from build123d import *

# Parameters (mm, degrees)
F0_W        = 50.8
F0_H        = 3.0988
F1_DEPTH    = 8.89
F3_R        = 1.778
F4_T1_DEPTH = 59.9449047052
F5_DEPTH    = 25.4


# Not quite as in the source:
# - a fillet or chamfer that OpenCascade refuses, or shapes differently, is made with other operations: its cross-section is extruded or revolved along the edge and cut away or added


with BuildPart() as f1:
    # F0 (on Top) → F1 (new body)
    with BuildSketch(Plane.XY):
        with Locations((0, 1.5494)):
            Rectangle(F0_W, F0_H)
    extrude(amount=F1_DEPTH)

    # F3
    f3_edges = [f1.edges().sort_by_distance(p)[0] for p in [
        (0, 3.0988, 8.89),
    ]]
    fillet(f3_edges, radius=F3_R)

    # F4: chamfer of 1.778 on 1 edges, made by hand

    # F4_s2 → F4_t1 (cut)
    with BuildSketch(Plane.YZ.offset(-29.9724523526)):
        Polygon((1.778, 8.89), (0, 7.112), (0, 8.89), align=None)
    extrude(amount=F4_T1_DEPTH, mode=Mode.SUBTRACT)

    # F2 (on face) → F5 (cut)
    with BuildSketch(Plane.XZ):
        Polygon((-22.225, 7.8332954744), (-21.6149113577, 8.89), (-22.8350886423, 8.89), align=None)
        Polygon((-12.6515878735, 8.89), (-14.0184121265, 8.89), (-13.335, 7.7062954744), align=None)
        Polygon((14.2383825791, 8.89), (12.4316174209, 8.89), (13.335, 7.3252954744), align=None)
        Polygon((22.225, 7.1982954744), (23.2017060633, 8.89), (21.2482939367, 8.89), align=None)
        Polygon((-3.6882643893, 8.89), (-5.2017356107, 8.89), (-4.445, 7.5792954744), align=None)
        Polygon((5.2750590949, 8.89), (3.6149409051, 8.89), (4.445, 7.4522954744), align=None)
    extrude(amount=-F5_DEPTH, mode=Mode.SUBTRACT)


solid = f1.part
Design review of the part built by this model. Coordinates are the model's own, in mm. Coordinates: 2 decimals unless noted, no trailing zeros. Loops run counter-clockwise (first coordinate to the right, second up) from the corner with the lowest first, then second, coordinate; pieces in that order, holes last. Notation, with made-up numbers: (-26, 16) -> (10, 16) arc R32 cw to (10, 50) -> close; hole circle Ø4 at (38, -36.75). An arc over 180 degrees is marked (long way). Use a Markdown table: item, result. Add a question column.
Item 1: We need section A-A, the plane x = 17.5. Write out the cut boundary in (y, z).
Item 2: We need section B-B, the plane y = 2.2. Write out the cut boundary in (x, z) (3 decimals), and give its area (3 significant figures).
Item 3: The part is to be moulded in two halves that separate along X. For faces 1 (the flat face through (-13.085, 1.779, 8.14)), 2 (the flat face through (-22, 1.82, 8.22)), 3 (the flat face through (-0.36, 0.88, 7.99)), 4 (the flat face through (25.4, 2, 4)), say which applies: +X half, -X half, draft (parallel to the pull), parting line (faces both ways), or undercut.
Item 4: Wall thickness on L1, parallel to Z at x = -22, y = 2.95; L2, parallel to Y at x = -4, z = 8; L3, parallel to Z at x = -23, y = 1.25: over which ranges is each line inside the solid? List them lowest first. Write a range as from..to.
Numbers:
| question | item | result |
|---|---|---|
| 1 | outline | (0, 0) -> (3.1, 0) -> (3.1, 7.11) arc R1.78 ccw to (1.73, 8.84) -> (0, 7.11) -> close |
| 2 | outline | (-25.4, 0) -> (25.4, 0) -> (25.4, 8.657) -> (23.067, 8.657) -> (22.225, 7.198) -> (21.383, 8.657) -> (14.104, 8.657) -> (13.335, 7.325) -> (12.566, 8.657) -> (5.141, 8.657) -> (4.445, 7.452) -> (3.749, 8.657) -> (-3.823, 8.657) -> (-4.445, 7.579) -> (-5.067, 8.657) -> (-12.786, 8.657) -> (-13.335, 7.706) -> (-13.884, 8.657) -> (-21.749, 8.657) -> (-22.225, 7.833) -> (-22.701, 8.657) -> (-25.4, 8.657) -> close |
| 2 | area | 435 mm^2 |
| 3 | face 1 | undercut |
| 3 | face 2 | undercut |
| 3 | face 3 | draft |
| 3 | face 4 | +X half |
| 4 | L1 | z = 0..7.82 |
| 4 | L2 | y = 0.89..2.86 |
| 4 | L3 | z = 0..8.36 |
